from build123d import *

# Parameters (mm, degrees)
SKETCH1_W           = 15
SKETCH1_H           = 36
BOSS_EXTRUDE1_DEPTH = 80
SKETCH2_R           = 6.5
CUT_EXTRUDE1_DEPTH  = 321


with BuildPart() as part:
    # Sketch1 → Boss-Extrude1 (new body)
    with BuildSketch(Plane(origin=(0, 0, 0), x_dir=(0, 0, -1), z_dir=(1, 0, 0))):
        with Locations((42.5, 38)):
            Rectangle(SKETCH1_W, SKETCH1_H)
        Polygon((320, 56), (310, 56), (310, 20), (10, 20), (10, 68), (0, 68), (0, 20), (0, 0), (320, 0), (320, 20), align=None)
    extrude(amount=BOSS_EXTRUDE1_DEPTH)

    # Sketch2 → Cut-Extrude1 (cut, through all)
    with BuildSketch(Plane(origin=(0, 0, -320), x_dir=(-1, 0, 0), z_dir=(0, 0, -1))):
        with Locations((-40, 40)):
            Circle(SKETCH2_R)
    extrude(amount=-CUT_EXTRUDE1_DEPTH, mode=Mode.SUBTRACT)


solid = part.part
The model under review builds one solid part; all positions refer to its coordinate system, in mm. A direction names the side the tool comes from. Round coordinates to 2 decimals unless told otherwise and drop trailing zeros. Order: outer loops, then holes, each group sorted by start corner. A loop starts at its lowest first (then second) coordinate and runs counter-clockwise, first axis right, second up. Notation, with made-up numbers: (39.5, 44.25) -> (51.5, 44.25) arc R33 ccw to (51.5, 81.25) -> close; hole circle Ø8 at (66.25, -28). An arc over 180 degrees is marked (long way). Return JSON: item names as keys, results as strings.
1. For faces 4 (the face through (39, 28, -320)), 5 (the face through (39, 20, -182)), 6 (the face through (39, 56, -315)), list the 3-axis set-ups (+Z, -Z, +X, -X, +Y, -Y) from which the entire face can be reached by the end or side of a thin tool; tool diameter is ignored.
Answer block:
{"face 4": "-Z, +X, -X, +Y, -Y", "face 5": "+X, -X, +Y", "face 6": "-Z, +X, -X, +Y"}
2. Insertion check: P1, Ø15, axis at x = 40, y = 40, coming from the +Z side; P2, Ø1, axis at x = 20.5, z = -262, coming from the +Y side; P3, Ø16.5, axis at x = 37.5, z = -44.5, coming from the +Y side; P4, Ø11.5, axis at x = 40, y = 40, coming from the +Z side. Each pin has a flat end and moves straight along its axis. Give the tip position at first contact, or say it passes through.
Answer block:
{"P1": "stops at z = 0", "P2": "stops at y = 20", "P3": "stops at y = 56", "P4": "passes through"}
3. The part is to be moulded in two halves that separate along Y. For faces 1 (the face through (46.494, 40.286, -42.605)), 2 (the face through (39, 56, -42)), 3 (the face through (39, 30, -50)), say which applies: +Y half, -Y half, draft (parallel to the pull), parting line (faces both ways), or undercut.
Answer block:
{"face 1": "undercut", "face 2": "+Y half", "face 3": "draft"}
4. Take a section at D-D (x = 53). Write out the cut boundary in (y, z).
Answer block:
{"outline": "(0, -320) -> (56, -320) -> (56, -310) -> (20, -310) -> (20, -50) -> (56, -50) -> (56, -35) -> (20, -35) -> (20, -10) -> (68, -10) -> (68, 0) -> (0, 0) -> close"}
5. Take a section at C-C (z = -47). Write out the cut boundary in (x, y).
Answer block:
{"outline": "(0, 0) -> (80, 0) -> (80, 56) -> (0, 56) -> close; hole circle Ø13 at (40, 40)"}
6. For L1, parallel to Z at x = 67, y = 31.5; L2, parallel to Y at x = 55.5, z = -15; L3, parallel to Y at x = 40, z = -43, list the stretches that pass through material, from the lowest coordinate up. Write a range as [from, to].
Answer block:
{"L1": "z = [-320, -310], [-50, -35], [-10, 0]", "L2": "y = [0, 20]", "L3": "y = [0, 33.5], [46.5, 56]"}
7. Take a section at A-A (y = 40). Write out the cut boundary in (x, z), then the cut area to 4 significant figures.
Answer block:
{"outline": "(0, -320) -> (33.5, -320) -> (33.5, -310) -> (0, -310) -> close; (0, -50) -> (33.5, -50) -> (33.5, -35) -> (0, -35) -> close; (0, -10) -> (33.5, -10) -> (33.5, 0) -> (0, 0) -> close; (46.5, -320) -> (80, -320) -> (80, -310) -> (46.5, -310) -> close; (46.5, -50) -> (80, -50) -> (80, -35) -> (46.5, -35) -> close; (46.5, -10) -> (80, -10) -> (80, 0) -> (46.5, 0) -> close", "area": "2,345 mm²"}
8. Take a section at B-B (x = 40). Write out the cut boundary in (y, z).
Answer block:
{"outline": "(0, -320) -> (33.5, -320) -> (33.5, -310) -> (20, -310) -> (20, -50) -> (33.5, -50) -> (33.5, -35) -> (20, -35) -> (20, -10) -> (33.5, -10) -> (33.5, 0) -> (0, 0) -> close; (46.5, -320) -> (56, -320) -> (56, -310) -> (46.5, -310) -> close; (46.5, -50) -> (56, -50) -> (56, -35) -> (46.5, -35) -> close; (46.5, -10) -> (68, -10) -> (68, 0) -> (46.5, 0) -> close"}
